```python
from build123d import *

# Parameters (mm, degrees)
SKETCH1_W           = 5.08
SKETCH1_H           = 3.81
BOSS_EXTRUDE1_DEPTH = 5.08
CUT_EXTRUDE1_DEPTH  = 5.08


with BuildPart() as part:
    # Sketch1 → Boss-Extrude1 (new body)
    with BuildSketch(Plane(origin=(0, 0, 0), x_dir=(1, 0, 0), z_dir=(0, 1, 0))):
        Polygon((-41.626929972, -5.1367648), (-9.740013168, -23.5466848), (22.146903635, -5.1367648), (22.146903635, 31.6830752), (-9.740013168, 50.0929952), (-41.626929972, 31.6830752), align=None)
        Polygon((-15.784801205, 36.4430352), (-13.244801205, 32.043626149), (-16.544357993, 30.138626149), (-19.084357993, 34.5380352), align=None, mode=Mode.SUBTRACT)
        with Locations((-30.288111869, 17.7181552)):
            Rectangle(SKETCH1_W, SKETCH1_H, mode=Mode.SUBTRACT)
        with Locations((-30.288111869, 8.8281552)):
            Rectangle(SKETCH1_W, SKETCH1_H, mode=Mode.SUBTRACT)
        Polygon((-26.783323833, 30.0930352), (-24.243323833, 25.693626149), (-20.943767044, 27.598626149), (-23.483767044, 31.9980352), align=None, mode=Mode.SUBTRACT)
        Polygon((7.303297496, 30.0930352), (4.763297496, 25.693626149), (1.463740708, 27.598626149), (4.003740708, 31.9980352), align=None, mode=Mode.SUBTRACT)
        Polygon((-3.695225132, 36.4430352), (-6.235225132, 32.043626149), (-2.935668344, 30.138626149), (-0.395668344, 34.5380352), align=None, mode=Mode.SUBTRACT)
        with Locations((10.808085532, 8.8281552)):
            Rectangle(SKETCH1_W, SKETCH1_H, mode=Mode.SUBTRACT)
        with Locations((10.808085532, 17.7181552)):
            Rectangle(SKETCH1_W, SKETCH1_H, mode=Mode.SUBTRACT)
        Polygon((-3.695225132, -9.8967248), (-6.235225132, -5.497315749), (-2.935668344, -3.592315749), (-0.395668344, -7.9917248), align=None, mode=Mode.SUBTRACT)
        Polygon((7.303297496, -3.5467248), (4.763297496, 0.852684251), (1.463740708, -1.052315749), (4.003740708, -5.4517248), align=None, mode=Mode.SUBTRACT)
        Polygon((-26.783323833, -3.5467248), (-24.243323833, 0.852684251), (-20.943767044, -1.052315749), (-23.483767044, -5.4517248), align=None, mode=Mode.SUBTRACT)
        Polygon((-15.784801205, -9.8967248), (-13.244801205, -5.497315749), (-16.544357993, -3.592315749), (-19.084357993, -7.9917248), align=None, mode=Mode.SUBTRACT)
    extrude(amount=BOSS_EXTRUDE1_DEPTH)

    # Sketch2 → Cut-Extrude1 (cut)
    with BuildSketch(Plane(origin=(0, 5.08, 0), x_dir=(1, 0, 0), z_dir=(0, 1, 0))):
        Polygon((-12.280013168, 20.8931552), (-9.740013168, 20.8931552), (-7.200013168, 20.8931552), (-7.200013168, 15.8131552), (-2.120013168, 15.8131552), (-2.120013168, 13.2731552), (-2.120013168, 10.7331552), (-7.200013168, 10.7331552), (-7.200013168, 5.6531552), (-9.740013168, 5.6531552), (-12.280013168, 5.6531552), (-12.280013168, 10.7331552), (-17.360013168, 10.7331552), (-17.360013168, 13.2731552), (-17.360013168, 15.8131552), (-12.280013168, 15.8131552), align=None)
    extrude(amount=-CUT_EXTRUDE1_DEPTH, mode=Mode.SUBTRACT)


solid = part.part
```
Design review of the part built by this model. Coordinates are the model's own, in mm. A direction names the side the tool comes from. Round coordinates to 2 decimals unless told otherwise and drop trailing zeros. Order: outer loops, then holes, each group sorted by start corner. A loop starts at its lowest first (then second) coordinate and runs counter-clockwise, first axis right, second up. Notation, with made-up numbers: (2, 60) - (15, 60) arc R22 ccw to (15, 70) - close; hole circle Ø8 at (7.25, -37.5). An arc over 180 degrees is marked (long way). One line per question, with ' | ' between items.
Item 1: Machinability: for faces 1 (the face through (-17.46, 2.5, 8.93)), 2 (the face through (-25.46, 2.504, -41.017)), which of the approach directions +Z, -Z, +X, -X, +Y, -Y give a long, thin tool a straight path to every point of the face, cutting with its end or side? Answer none if there is none.
Checks:
face 1: +Y, -Y | face 2: -Z, -X, +Y, -Y
Item 2: Take a section at B-B, the plane x = -22.5. Write out the cut boundary in (y, z).
Checks:
outline: (0, -42.73) - (5.08, -42.73) - (5.08, -30.29) - (0, -30.29) - close; (0, -26.7) - (5.08, -26.7) - (5.08, 0.15) - (0, 0.15) - close; (0, 3.75) - (5.08, 3.75) - (5.08, 16.18) - (0, 16.18) - close
Item 3: Wall thickness on line 1 (X direction, y = 0.8, z = -18.5); line 2 (X direction, y = 1.1, z = -13); line 3 (Z direction, x = 9.5, y = 1.95): over which ranges is each line inside the solid? List them lowest first. Write a range as [from, to].
Checks:
line 1: [-41.63, -32.83], [-27.75, -12.28], [-7.2, 8.27], [13.35, 22.15] | line 2: [-41.63, -17.36], [-2.12, 22.15] | line 3: [-38.98, -19.62], [-15.81, -10.73], [-6.92, 12.44]
Item 4: For P1, Ø3, axis at x = -33.5, z = -37.5, coming from the +Y side; P2, Ø1.5, axis at x = -15.5, y = 1.5, coming from the +Z side; P3, Ø1.5, axis at x = -30, y = 1.5, coming from the +Z side; P4, Ø2.5, axis at x = 12, y = 2.5, coming from the -Z side, all flat-tipped, find the tip position at first contact; note any pin that passes through.
Checks:
P1: y = 5.08 | P2: z = 20.65 | P3: z = 12.28 | P4: z = -38.26
Item 5: Draft analysis for pull direction Y (two halves, no side actions). For faces 3 (the face through (22.147, 3, -13)), 4 (the face through (-17, 5.08, -6)), state which applies: +Y half, -Y half, draft (parallel to the pull), parting line (faces both ways), or undercut.
Checks:
face 3: draft | face 4: +Y half
Item 6: Take a section at D-D, the plane z = -33.5. Write out the cut boundary in (x, y).
Checks:
outline: (-38.48, 0) - (-18.49, 0) - (-18.49, 5.08) - (-38.48, 5.08) - close; (-14.09, 0) - (-5.39, 0) - (-5.39, 5.08) - (-14.09, 5.08) - close; (-0.99, 0) - (19, 0) - (19, 5.08) - (-0.99, 5.08) - close
Item 7: Take a section at C-C, the plane y = 1.5. Give the number of separate pieces and of enclosed holes in the cut face, then the cut area to 3 significant figures.
Checks:
separate pieces: 1 | enclosed holes: 13 | area: 3,160 mm²
Item 8: Take a section at A-A, the plane z = -17.5. Write out the cut boundary in (x, y), then the cut area to 3 significant figures.
Checks:
outline: (-41.63, 0) - (-32.83, 0) - (-32.83, 5.08) - (-41.63, 5.08) - close; (-27.75, 0) - (-12.28, 0) - (-12.28, 5.08) - (-27.75, 5.08) - close; (-7.2, 0) - (8.27, 0) - (8.27, 5.08) - (-7.2, 5.08) - close; (13.35, 0) - (22.15, 0) - (22.15, 5.08) - (13.35, 5.08) - close | area: 247 mm²
